from build123d import *

# Parameters (mm, degrees)
SKETCH_1_W                         = 50
SKETCH_1_H                         = 7
EXTRUDE_1_DEPTH                    = 10
CUT_EXTRUDE_2_DEPTH                = 7.5
CHAMFER_2_SIZE                     = 0.6
CHAMFER_2_SIZE2                    = 3.402769092
CUT_EXTRUDE_1775_DEPTH             = 28.152347965
CUT_EXTRUDE_1775_DEPTH_BACK        = 28.152347965
CUT_EXTRUDE_1975_REACH             = 29.152
CUT_EXTRUDE_1975_DIRECTION_2_REACH = 29.152


with BuildPart() as part:
    # Эскиз1 → Бобышка-Вытянуть1 (new body)
    with BuildSketch(Plane(origin=(0, 66.754264805, 0), x_dir=(-1, 0, 0), z_dir=(0, 0, 1))):
        with Locations((0, 66.754264805)):
            Rectangle(SKETCH_1_W, SKETCH_1_H)
    extrude(amount=EXTRUDE_1_DEPTH)

    # Эскиз4 → Вырез-Вытянуть2 (cut)
    with BuildSketch(Plane(origin=(0, 66.754264805, 10), x_dir=(-1, 0, 0), z_dir=(0, 0, 1))):
        Polygon((-20.9, 67.204264805), (-12.5, 67.204264805), (-11.75, 68.404264805), (-11, 67.204264805), (11, 67.204264805), (11.75, 68.404264805), (12.5, 67.204264805), (20.9, 67.204264805), (20.9, 66.304264805), (-20.9, 66.304264805), align=None)
    extrude(amount=-CUT_EXTRUDE_2_DEPTH, mode=Mode.SUBTRACT)

    # Фаска2
    chamfer_2_edges = [part.edges().sort_by_distance(p)[0] for p in [
        (11.375, -1.05, 2.5),
        (-11.375, -1.05, 2.5),
        (-12.125, -1.05, 2.5),
        (12.125, -1.05, 2.5),
    ]]
    chamfer_2_side = [part.faces().sort_by_distance(p)[0] for p in [
        (0, -0.038812785, 2.5),
    ]]
    chamfer(chamfer_2_edges, length=CHAMFER_2_SIZE, length2=CHAMFER_2_SIZE2, reference=chamfer_2_side[0])

    # Эскиз5 → Cut-Extrude 1775 (cut, two sides: drawn at the far end of the back side and taken through both)
    with BuildSketch(Plane(origin=(0, 0, 0), x_dir=(0, 0, -1), z_dir=(1, 0, 0)).offset(-CUT_EXTRUDE_1775_DEPTH_BACK)):
        with BuildLine():
            Line((-10, -1), (-10, 3.5))
            Line((-10, 3.5), (-5.644148579, 3.5))
            Line((-5.644148579, 3.5), (-8.361695911, 1.597152873))
            ThreePointArc((-8.361695911, 1.597152873), (-9.442167509, 0.463418829), (-10, -1))
        make_face()
    extrude(amount=CUT_EXTRUDE_1775_DEPTH + CUT_EXTRUDE_1775_DEPTH_BACK, mode=Mode.SUBTRACT)

    # Cut-Extrude 1975: up to this face of the body (flat: up to its plane)
    cut_extrude_1975_end = Plane(part.part.faces().sort_by_distance((-20.9, -0.004333952, 6.091884202))[0])
    # Эскиз6 → Cut-Extrude 1975 (cut, up to the picked face)
    with BuildSketch(Plane(origin=(0, 0, 0), x_dir=(0, 0, -1), z_dir=(1, 0, 0)), mode=Mode.PRIVATE) as cut_extrude_1975_sk1:
        with BuildLine():
            Line((-8.00005385, 1.85037737), (-10.83265057, -0.133028206))
            ThreePointArc((-10.83265057, -0.133028206), (-8.786352952, -0.894909941), (-8.147597927, 1.193101011))
            ThreePointArc((-8.147597927, 1.193101011), (-8.201124989, 1.550315037), (-8.00005385, 1.85037737))
        make_face()
    cut_extrude_1975_tool1 = split(extrude(cut_extrude_1975_sk1.sketch, amount=-CUT_EXTRUDE_1975_REACH, mode=Mode.PRIVATE), bisect_by=cut_extrude_1975_end, keep=Keep.BOTH, mode=Mode.PRIVATE)
    add(cut_extrude_1975_tool1.solids().sort_by(Axis((0, 0.082385, 9.170045), (-1, 0, 0)))[0], mode=Mode.SUBTRACT)

    # Cut-Extrude 1975 direction 2: up to this face of the body (flat: up to its plane)
    cut_extrude_1975_direction_2_end = Plane(part.part.faces().sort_by_distance((20.9, -0.004333952, 6.091884202))[0])
    # Эскиз6 → Cut-Extrude 1975 direction 2 (cut, up to the picked face)
    with BuildSketch(Plane(origin=(0, 0, 0), x_dir=(0, 0, -1), z_dir=(1, 0, 0)), mode=Mode.PRIVATE) as cut_extrude_1975_direction_2_sk1:
        with BuildLine():
            Line((-8.00005385, 1.85037737), (-10.83265057, -0.133028206))
            ThreePointArc((-10.83265057, -0.133028206), (-8.786352952, -0.894909941), (-8.147597927, 1.193101011))
            ThreePointArc((-8.147597927, 1.193101011), (-8.201124989, 1.550315037), (-8.00005385, 1.85037737))
        make_face()
    cut_extrude_1975_direction_2_tool1 = split(extrude(cut_extrude_1975_direction_2_sk1.sketch, amount=CUT_EXTRUDE_1975_DIRECTION_2_REACH, mode=Mode.PRIVATE), bisect_by=cut_extrude_1975_direction_2_end, keep=Keep.BOTH, mode=Mode.PRIVATE)
    add(cut_extrude_1975_direction_2_tool1.solids().sort_by(Axis((0, 0.082385, 9.170045), (1, 0, 0)))[0], mode=Mode.SUBTRACT)


solid = part.part
Read the model definition and answer for the solid it produces. Units are mm, in the model's axes. A direction names the side the tool comes from. Give positions to 0.01 mm unless a question says otherwise; leave off trailing zeros. Write each loop counter-clockwise with the first axis right and the second up, starting at its lowest first coordinate (ties: lowest second). Pieces come first, ordered by that corner, then holes. Notation, with made-up numbers: (88, -39) - (106, -39) arc R10 cw to (106, -35) - close; hole circle Ø10 at (43, 69). An arc over 180 degrees is marked (long way). Use CSV: the item, a comma, the result in double quotes. Start each with the question number.
Item 1: The part is cut by section B-B, the plane x = -16. Give the vertices of the cut face in (y, z) (3 decimals).
Item 2: Consider line 1 (Y direction, x = -10, z = 3); line 2 (X direction, y = -1.25, z = 7.75). Determine where each line is inside the solid, lowest interval first.
Item 3: The part is cut by section A-A, the plane z = 3.25. Give the vertices of the cut face in (x, y), and give its area (3 significant figures).
Item 4: The part is cut by section D-D, the plane z = 7.5. Give the vertices of the cut face in (x, y).
Item 5: For faces 4 (the cylindrical face through (-0.16, -0.996, 9.05)), 5 (the flat face through (11.49, -0.8, 4.6)), 6 (the flat face through (-0.35, 2.562, 6.984)), determine the directions among +Z, -Z, +X, -X, +Y, -Y from which every point of the face is accessible in a straight line to the end or side of a thin tool.
Item 6: The part is cut by section C-C, the plane x = 22. Give the vertices of the cut face in (y, z) (3 decimals).
Item 7: The mould has two halves that part along Y. Classify faces 1 (the flat face through (25, 0, 5)), 2 (the flat face through (0, 3.5, 3)), 3 (the flat face through (0, 0, 2.5)): pulls with the +Y half, pulls with the -Y half, needs draft (parallel to the pull), parting line crosses it, or undercut.
Item 8: A flat-ended cylindrical pin translates along its axis: P1, Ø1.1, axis at x = -5.5, y = 0, coming from the +Z side. Find the tip coordinate at first contact, or state that the pin passes through.
Taken from the geometry:
1,outline,"(-3.5, 0) - (3.5, 0) - (3.5, 5.644) - (1.85, 8) arc R0.5 ccw to (1.193, 8.148) arc R1.5 cw to (0.45, 7.951) - (0.45, 2.5) - (-0.45, 2.5) - (-0.45, 8.251) arc R1.5 cw to (-0.949, 9.991) arc R3.969 ccw to (-1, 10) - (-3.5, 10) - close"
2,line 1,"-3.5 to -0.45, 0.45 to 3.5"
2,line 2,"-25 to -12, -11.5 to 11.5, 12 to 25"
3,outline,"(-25, -3.5) - (25, -3.5) - (25, 3.5) - (-25, 3.5) - close; hole (-20.9, -0.45) - (-11.95, -0.45) - (-11.75, -0.77) - (-11.55, -0.45) - (11.55, -0.45) - (11.75, -0.77) - (11.95, -0.45) - (20.9, -0.45) - (20.9, 0.45) - (-20.9, 0.45) - close"
3,area,"312 mm2"
4,outline,"(-25, -3.5) - (25, -3.5) - (25, 2.2) - (-25, 2.2) - close; hole (-20.9, -0.45) - (-12.5, -0.45) - (-11.75, -1.65) - (-11, -0.45) - (11, -0.45) - (11.75, -1.65) - (12.5, -0.45) - (20.9, -0.45) - (20.9, 0.45) - (-20.9, 0.45) - close"
5,face 4,"+Y"
5,face 5,"+Z"
5,face 6,"+Z, +X, -X, +Y"
6,outline,"(-3.5, 0) - (3.5, 0) - (3.5, 5.644) - (1.597, 8.362) arc R3.969 ccw to (-1, 10) - (-3.5, 10) - close"
7,face 1,"needs draft"
7,face 2,"pulls with the +Y half"
7,face 3,"undercut"
8,P1,"z = 8.33"
